Work out the finished part from the listing and answer in its coordinate system (mm). A direction names the side the tool comes from. Round coordinates to 2 decimals unless told otherwise and drop trailing zeros. Order: outer loops, then holes, each group sorted by start corner. A loop starts at its lowest first (then second) coordinate and runs counter-clockwise, first axis right, second up. Notation, with made-up numbers: (-4, 34) - (44, 34) arc R13 cw to (44, 51) - close; hole circle Ø4 at (6.25, -6.5). An arc over 180 degrees is marked (long way). Use CSV: the item, a comma, the result in double quotes.
from build123d import *

# Parameters (mm, degrees)
SKETCH1_R           = 3.7592
SKETCH1_W           = 1.5875
SKETCH1_H           = 1.3208
BOSS_EXTRUDE1_DEPTH = 1.5875
CUT_EXTRUDE1_REACH  = 32.926


with BuildPart() as part:
    # Sketch1 → Boss-Extrude1 (new body)
    # profile 1 of 6: a face of its own
    with BuildSketch(Plane.XY):
        with BuildLine():
            Line((2.54, 21.59), (9.525, 21.59))
            Line((9.525, 21.59), (9.525, -3.81))
            Line((9.525, -3.81), (-10.16, -3.81))
            Line((-10.16, -3.81), (-10.16, 8.89))
            ThreePointArc((-10.16, 8.89), (-6.440256121, 17.870256121), (2.54, 21.59))
        make_face()
        Circle(SKETCH1_R, mode=Mode.SUBTRACT)
        with BuildLine():
            ThreePointArc((-3.82905, 11.642311449), (-7.874, 9.144), (-3.82905, 6.645688551))
            ThreePointArc((-3.82905, 6.645688551), (4.572, 9.144), (-3.82905, 11.642311449))
        make_face(mode=Mode.SUBTRACT)
    # profile 2 of 6: a face of its own
    with BuildSketch(Plane.XY):
        with Locations((-10.95375, -1.5494)):
            Rectangle(SKETCH1_W, SKETCH1_H)
    # profile 3 of 6: a face of its own
    with BuildSketch(Plane.XY):
        with Locations((10.31875, 17.1704)):
            Rectangle(SKETCH1_W, SKETCH1_H)
    # profile 4 of 6: a face of its own
    with BuildSketch(Plane.XY):
        with Locations((10.31875, 0.6604)):
            Rectangle(SKETCH1_W, SKETCH1_H)
    # profile 5 of 6: a face of its own
    with BuildSketch(Plane.XY):
        with BuildLine():
            ThreePointArc((-10.16, 8.89), (-9.508277885, 12.906092628), (-7.62, 16.51))
            Line((-7.62, 16.51), (-17.51946076, 16.51))
            Line((-17.51946076, 16.51), (-22.084921519, 15.486982224))
            Line((-22.084921519, 15.486982224), (-22.084921519, 13.081))
            Line((-22.084921519, 13.081), (-22.084921519, 4.699))
            Line((-22.084921519, 4.699), (-22.084921519, 2.212007412))
            Line((-22.084921519, 2.212007412), (-10.16, 4.318))
            Line((-10.16, 4.318), (-10.16, 8.89))
        make_face()
    # profile 6 of 6: a face of its own
    with BuildSketch(Plane.XY):
        with BuildLine():
            ThreePointArc((-10.16, 8.89), (-9.508277885, 12.906092628), (-7.62, 16.51))
            Line((-7.62, 16.51), (-17.51946076, 16.51))
            Line((-17.51946076, 16.51), (-22.084921519, 15.486982224))
            Line((-22.084921519, 15.486982224), (-22.084921519, 13.081))
            Line((-22.084921519, 13.081), (-22.084921519, 4.699))
            Line((-22.084921519, 4.699), (-22.084921519, 2.212007412))
            Line((-22.084921519, 2.212007412), (-10.16, 4.318))
            Line((-10.16, 4.318), (-10.16, 8.89))
        make_face()
    extrude(amount=BOSS_EXTRUDE1_DEPTH)

    # Sketch2 → Cut-Extrude1 (cut, up to next)
    with BuildSketch(Plane.XY.offset(1.5875), mode=Mode.PRIVATE) as cut_extrude1_sk1:
        Polygon((6.223, -0.0889), (6.223, -3.81), (9.525, -3.81), (9.525, -3.0226), (9.525, -0.9144), (9.525, -0.0889), align=None)
    cut_extrude1_tool1 = extrude(cut_extrude1_sk1.sketch, amount=-CUT_EXTRUDE1_REACH, mode=Mode.PRIVATE) & part.part
    # Sketch2 → Cut-Extrude1 (cut, up to next)
    with BuildSketch(Plane.XY.offset(1.5875), mode=Mode.PRIVATE) as cut_extrude1_sk2:
        Polygon((9.525, 18.6944), (9.525, 20.8026), (9.525, 21.59), (6.223, 21.59), (6.223, 17.8689), (9.525, 17.8689), align=None)
    cut_extrude1_tool2 = extrude(cut_extrude1_sk2.sketch, amount=-CUT_EXTRUDE1_REACH, mode=Mode.PRIVATE) & part.part
    add(cut_extrude1_tool1.solids().sort_by_distance((7.874, -1.94945, 1.5875))[0], mode=Mode.SUBTRACT)
    add(cut_extrude1_tool2.solids().sort_by_distance((7.874, 19.72945, 1.5875))[0], mode=Mode.SUBTRACT)


solid = part.part
(1) Find section D-D (z = 0.35). State how many separate pieces and enclosed holes the cut face has, and give its area (3 significant figures).
Findings below:
separate pieces,"1"
enclosed holes,"2"
area,"482 mm²"
(2) Find section B-B (y = 8). Determine the outline of the cut face in (x, z) (1 decimal).
Findings below:
outline,"(-22.1, 0) - (-7.6, 0) - (-7.6, 1.6) - (-22.1, 1.6) - close; (4.4, 0) - (9.5, 0) - (9.5, 1.6) - (4.4, 1.6) - close"
(3) Each of these flat-tipped pins is pushed along its axis until it touches: pin 1 (0.8 mm diameter, centred on x = -11.5, z = 0.5, fed in from +Y); pin 2 (0.8 mm diameter, centred on x = 10.5, z = 1, fed in from +Y); pin 3 (0.5 mm diameter, centred on y = -2.5, z = 0.5, fed in from -X). Where does it stop, or does it pass through?
Findings below:
pin 1,"stops at y = 16.51"
pin 2,"stops at y = 17.83"
pin 3,"stops at x = -10.16"
(4) Find section A-A (x = -5.08). Determine the outline of the cut face in (y, z), and give its area (3 significant figures).
Findings below:
outline,"(-3.81, 0) - (6.35, 0) - (6.35, 1.59) - (-3.81, 1.59) - close; (11.94, 0) - (19.05, 0) - (19.05, 1.59) - (11.94, 1.59) - close"
area,"27.4 mm²"
(5) Find section C-C (x = -1). Determine the outline of the cut face in (y, z), and give its area (3 significant figures).
Findings below:
outline,"(-3.81, 0) - (-3.62, 0) - (-3.62, 1.59) - (-3.81, 1.59) - close; (3.62, 0) - (4.68, 0) - (4.68, 1.59) - (3.62, 1.59) - close; (13.61, 0) - (21.09, 0) - (21.09, 1.59) - (13.61, 1.59) - close"
area,"13.9 mm²"
(6) Find the intervals of material crossed by L1, parallel to Y at x = -2.5, z = 0.25; L2, parallel to Y at x = 2, z = 0.35; L3, parallel to X at y = 9.25, z = 0.65 (3 decimals), in increasing order. Write a range as from..to.
Findings below:
L1,"y = -3.81..-2.81, 2.81..5.32, 12.97..20.55"
L2,"y = -3.81..-3.18, 3.18..5.03, 13.26..21.58"
L3,"x = -22.085..-7.872, 4.571..9.525"
(7) For faces 1 (the flat face through (-11.747, -2, 1)), 2 (the flat face through (6.223, -2, 1)), 3 (the flat face through (-10.16, 2, 1)), 4 (the flat face through (9.525, 9, 1)), determine the directions among +Z, -Z, +X, -X, +Y, -Y from which every point of the face is accessible in a straight line to the end or side of a thin tool.
Findings below:
face 1,"+Z, -Z, -X, -Y"
face 2,"+Z, -Z, +X, -Y"
face 3,"+Z, -Z"
face 4,"+Z, -Z, +X"
